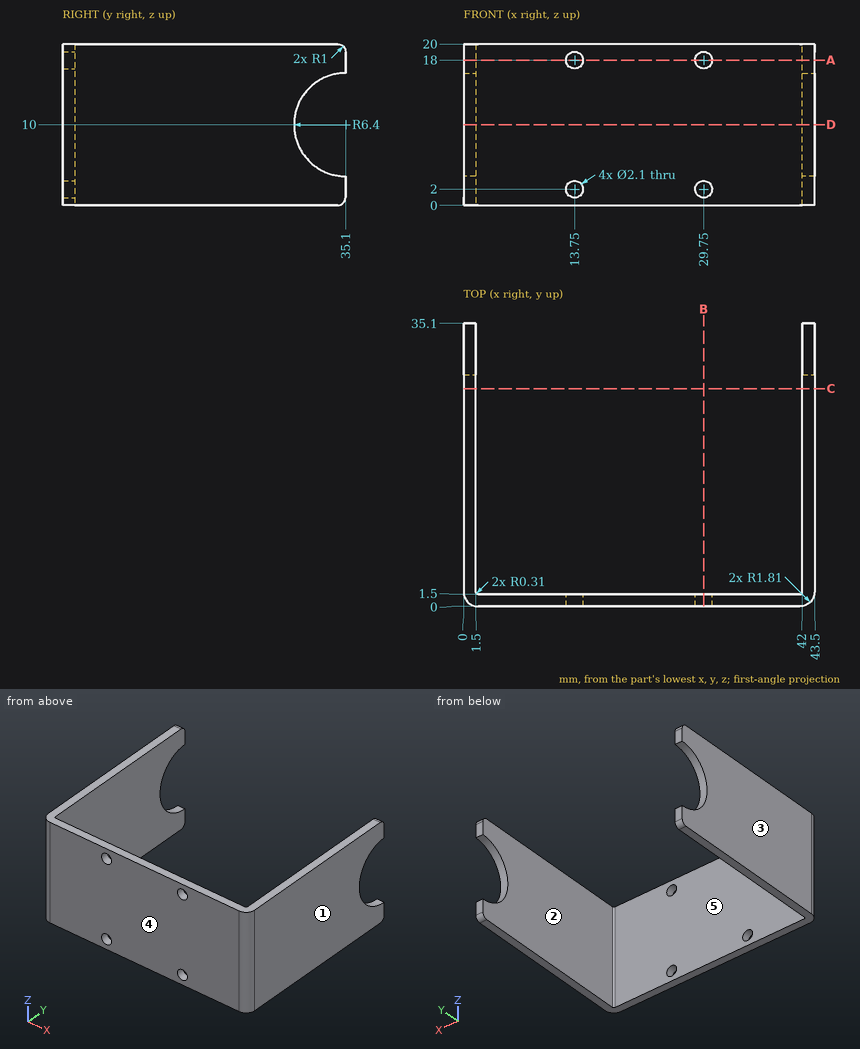
Job drawing, mm, ordinate dimensions from the low corner. One solid piece. A direction names the side the tool comes from. Round coordinates to 2 decimals unless told otherwise and drop trailing zeros. Write each loop counter-clockwise with the first axis right and the second up, starting at its lowest first coordinate (ties: lowest second). Pieces come first, ordered by that corner, then holes.
1) Mould opens along X. For the marked faces 3, 4 and 5 say: +X half, -X half, draft (parallel to the pull), parting line (faces both ways), or undercut.
2) Band-saw the part on D-D, the plane z = 10. List the corners of the cut face in (x, y), and give its area (3 significant figures).
3) Band-saw the part on B-B, the plane x = 29.75. List the corners of the cut face in (y, z), and give its area (3 significant figures).
4) Band-saw the part on A-A, the plane z = 18. List the corners of the cut face in (x, y).
5) Pin check, flat tip, straight feed: pin 1 (12 mm diameter, centred on x = 30.5, z = 12, fed in from +Y). Stop position of the tip, or through.
6) 3-axis set-ups, long thin cutter, end or side, ignore diameter. For the marked faces 1 and 2: which of +Z, -Z, +X, -X, +Y, -Y reach the whole face in a straight line?
7) Drill centre lines: probe 1 along Z at (x, y) = (13.75, 0.85); probe 2 along X at (y, z) = (4, 5); probe 3 along Z at (x, y) = (13, 1). Where is each one in solid material? Low to high.
8) Band-saw the part on C-C, the plane y = 27. List the corners of the cut face in (x, z).
Ans:
1. face 3: -X half
1. face 4: draft
1. face 5: undercut
2. outline: (0, 1.81) arc R1.81 ccw to (1.81, 0) - (41.69, 0) arc R1.81 ccw to (43.5, 1.81) - (43.5, 28.7) - (42, 28.7) - (42, 1.81) arc R0.31 cw to (41.69, 1.5) - (1.81, 1.5) arc R0.31 cw to (1.5, 1.81) - (1.5, 28.7) - (0, 28.7) - close
2. area: 145 mm2
3. outline: (0, 0) - (1.5, 0) - (1.5, 0.95) - (0, 0.95) - close; (0, 3.05) - (1.5, 3.05) - (1.5, 16.95) - (0, 16.95) - close; (0, 19.05) - (1.5, 19.05) - (1.5, 20) - (0, 20) - close
3. area: 23.7 mm2
4. outline: (0, 1.81) arc R1.81 ccw to (1.81, 0) - (12.7, 0) - (12.7, 1.5) - (1.81, 1.5) arc R0.31 cw to (1.5, 1.81) - (1.5, 35.1) - (0, 35.1) - close; (14.8, 0) - (28.7, 0) - (28.7, 1.5) - (14.8, 1.5) - close; (30.8, 0) - (41.69, 0) arc R1.81 ccw to (43.5, 1.81) - (43.5, 35.1) - (42, 35.1) - (42, 1.81) arc R0.31 cw to (41.69, 1.5) - (30.8, 1.5) - close
5. pin 1: stops at y = 1.5
6. face 1: +Z, -Z, +X, +Y, -Y
6. face 2: +Z, -Z, +Y
7. probe 1: z = 0 to 0.95, 3.05 to 16.95, 19.05 to 20
7. probe 2: x = 0 to 1.5, 42 to 43.5
7. probe 3: z = 0 to 1.27, 2.73 to 17.27, 18.73 to 20
8. outline: (0, 0) - (1.5, 0) - (1.5, 20) - (0, 20) - close; (42, 0) - (43.5, 0) - (43.5, 20) - (42, 20) - close
